```python
from build123d import *

# Parameters (mm, degrees)
MAIN_DEPTH         = 25
SKETCH2_R          = 2
SKETCH2_R_2        = 1.5
HOLES_DEPTH        = 7.5
SKETCH3_W          = 10
SKETCH3_H          = 2.5
CUT_EXTRUDE2_DEPTH = 11


with BuildPart() as part:
    # Sketch1 → Main (new body, symmetric)
    with BuildSketch(Plane.XY):
        Polygon((-5, 0), (5, 0), (5, -5.5), (1.45, -5.5), (1.45, -6.5), (-1.45, -6.5), (-1.45, -5.5), (-5, -5.5), align=None)
    extrude(amount=MAIN_DEPTH, both=True)

    # Sketch2 → Holes (cut, through all)
    with BuildSketch(Plane(origin=(0, 0, 0), x_dir=(1, 0, 0), z_dir=(0, 1, 0))):
        with Locations((0, 20)):
            Circle(SKETCH2_R)
        with Locations((0, -20)):
            Circle(SKETCH2_R)
        Circle(SKETCH2_R_2)
    extrude(amount=-HOLES_DEPTH, mode=Mode.SUBTRACT)

    # Sketch3 → Cut-Extrude2 (cut, through all)
    with BuildSketch(Plane.ZY.offset(5)):
        with Locations((0, -1.25)):
            Rectangle(SKETCH3_W, SKETCH3_H)
    extrude(amount=-CUT_EXTRUDE2_DEPTH, mode=Mode.SUBTRACT)


solid = part.part
```
Build history of the part. All positions in model axes, mm. A direction names the side the tool comes from. Coordinates: 2 decimals unless noted, no trailing zeros. Write each loop counter-clockwise with the first axis right and the second up, starting at its lowest first coordinate (ties: lowest second). Pieces come first, ordered by that corner, then holes.
1. 3-axis set-ups, long thin cutter, end or side, ignore diameter. For faces 4 (the flat face through (-1.2, -2.5, -1.2)), 5 (the flat face through (3, -5.5, 0)), 6 (the flat face through (-1.45, -6, -9)), 7 (the flat face through (0, 0, -15)), 8 (the flat face through (0, -6.5, 10)): which of +Z, -Z, +X, -X, +Y, -Y reach the whole face in a straight line?
Answer block:
face 4: +X, -X, +Y
face 5: +Z, -Z, +X, -Y
face 6: +Z, -Z, -X, -Y
face 7: +Z, -Z, +X, -X, +Y
face 8: +Z, -Z, +X, -X, -Y
2. Band-saw the part on B-B, the plane x = 0. Give the cut face in (y, z).
Answer block:
outline: (-6.5, -25) - (0, -25) - (0, -22) - (-6.5, -22) - close; (-6.5, -18) - (0, -18) - (0, -5) - (-2.5, -5) - (-2.5, -1.5) - (-6.5, -1.5) - close; (-6.5, 1.5) - (-2.5, 1.5) - (-2.5, 5) - (0, 5) - (0, 18) - (-6.5, 18) - close; (-6.5, 22) - (0, 22) - (0, 25) - (-6.5, 25) - close
3. Band-saw the part on C-C, the plane y = -3. Give the cut face in (x, z).
Answer block:
outline: (-5, -25) - (5, -25) - (5, 25) - (-5, 25) - close; hole circle Ø4 at (0, -20); hole circle Ø4 at (0, 20); hole circle Ø3 at (0, 0)
4. Band-saw the part on A-A, the plane y = -1. Give the cut face in (x, z), and give its area (3 significant figures).
Answer block:
outline: (-5, -25) - (5, -25) - (5, -5) - (-5, -5) - close; (-5, 5) - (5, 5) - (5, 25) - (-5, 25) - close; hole circle Ø4 at (0, -20); hole circle Ø4 at (0, 20)
area: 375 mm2
5. Drop flat-ended pins along their axis: pin 1 (1.1 mm diameter, centred on y = -6, z = -11, fed in from +X); pin 2 (0.5 mm diameter, centred on y = -6, z = -23, fed in from +X); pin 3 (3 mm diameter, centred on x = 1, z = -2, fed in from +Y); pin 4 (2.5 mm diameter, centred on x = 0, z = 20, fed in from +Y). Give the stop position or say it passes through.
Answer block:
pin 1: stops at x = 5
pin 2: stops at x = 1.45
pin 3: stops at y = -2.5
pin 4: passes through
6. Pull direction X, two halves, no side cores. Call faces 1 (the flat face through (0, 0, 15)), 2 (the cylindrical face through (1.908, -3.204, 19.399)), 3 (the flat face through (-1.45, -6, 23)): released by +X, released by -X, zero draft, split by the parting line, or undercut.
Answer block:
face 1: zero draft
face 2: undercut
face 3: released by -X
7. Drill centre lines: probe 1 along Z at (x, y) = (0, -5.25); probe 2 along Z at (x, y) = (0, -1.25); probe 3 along X at (y, z) = (-4.5, -20). Where is each one in solid material? Low to high.
Answer block:
probe 1: z = -25 to -22, -18 to -1.5, 1.5 to 18, 22 to 25
probe 2: z = -25 to -22, -18 to -5, 5 to 18, 22 to 25
probe 3: x = -5 to -2, 2 to 5
8. Band-saw the part on D-D, the plane z = -20. Give the cut face in (x, y).
Answer block:
outline: (-5, -5.5) - (-2, -5.5) - (-2, 0) - (-5, 0) - close; (2, -5.5) - (5, -5.5) - (5, 0) - (2, 0) - close
